The model under review builds one solid part; all positions refer to its coordinate system, in mm. Face numbers are marked on the shaded views. A direction names the side the tool comes from. Coordinates: 2 decimals unless noted, no trailing zeros. Loops run counter-clockwise (first coordinate to the right, second up) from the corner with the lowest first, then second, coordinate; pieces in that order, holes last. Notation, with made-up numbers: (20, 14) - (38, 14) arc R19 cw to (38, 38) - close; hole circle Ø9 at (-10.5, 54.25). An arc over 180 degrees is marked (long way). One line per item, written item: value. Start each with the question number.
1. Mouldability with a two-part tool opening along X and no side actions: class the marked faces 1, 2 and 3 as +X half, -X half, draft (parallel to the pull), parting line (faces both ways), or undercut.
2. For the marked faces 4, 5 and 6, list the 3-axis set-ups (+Z, -Z, +X, -X, +Y, -Y) from which the entire face can be reached by the end or side of a thin tool; tool diameter is ignored.
3. To check wall thickness, follow line 1 (X direction, y = 2.3, z = 0); line 2 (X direction, y = 0.8, z = 0); line 3 (Y direction, x = -3.5, z = -4.5). State the ranges of each line that lie inside material, in increasing order.
4. Insertion check: P1, Ø3.5, axis at x = 0, z = 0, coming from the -Y side; P2, Ø0.7, axis at x = -0.5, y = 10, coming from the -Z side; P3, Ø2, axis at x = 3, y = 10.5, coming from the +Z side. Each pin has a flat end and moves straight along its axis. Give the tip position at first contact, or say it passes through.
5. We need section A-A, the plane x = 0. Give the boundary of the cut face in (y, z), then the cut area to 3 significant figures.
6. We need section D-D, the plane z = 10.25. Give the boundary of the cut face in (x, y), then the cut area to 3 significant figures.
7. We need section B-B, the plane y = 5.75. Give the boundary of the cut face in (x, z).
8. We need section C-C, the plane z = -2.5. Give the boundary of the cut face in (x, y), then the cut area to 3 significant figures.
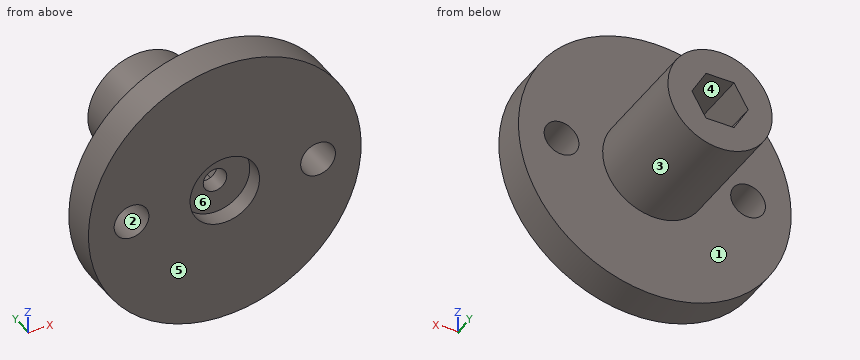
from build123d import *

# Parameters (mm, degrees)
SKETCH1_R           = 11.7729
SKETCH1_R_2         = 1.016
BOSS_EXTRUDE1_DEPTH = 3
SKETCH2_R           = 1.5
CUT_EXTRUDE1_DEPTH  = 17.917516036
SKETCH4_R           = 3
CUT_EXTRUDE3_DEPTH  = 1.5
SKETCH6_R           = 4.5
BOSS_EXTRUDE4_DEPTH = 10
CUT_EXTRUDE4_DEPTH  = 20.421697887


with BuildPart() as part:
    # Sketch1 → Boss-Extrude1 (new body)
    with BuildSketch(Plane(origin=(0, 0, 0), x_dir=(1, 0, 0), z_dir=(0, 1, 0))):
        with Locations(Location((0, 0, 0), (0, 0, 270))):
            Circle(SKETCH1_R)
        with Locations(Location((0, 0, 0), (0, 0, 270))):
            Circle(SKETCH1_R_2, mode=Mode.SUBTRACT)
    extrude(amount=BOSS_EXTRUDE1_DEPTH)

    # Sketch2 → Cut-Extrude1 (cut, through all)
    with BuildSketch(Plane(origin=(0, 3, 0), x_dir=(1, 0, 0), z_dir=(0, 1, 0))):
        with Locations(Location((8.0518, 0, 0), (0, 0, 270))):
            Circle(SKETCH2_R)
        with Locations(Location((-8.0518, 0, 0), (0, 0, 270))):
            Circle(SKETCH2_R)
    extrude(amount=-CUT_EXTRUDE1_DEPTH, mode=Mode.SUBTRACT)

    # Sketch4 → Cut-Extrude3 (cut)
    with BuildSketch(Plane.XZ):
        with Locations(Location((0, 0, 0), (0, 0, 270))):
            Circle(SKETCH4_R)
    extrude(amount=-CUT_EXTRUDE3_DEPTH, mode=Mode.SUBTRACT)

    # Sketch6 → Boss-Extrude4 (add)
    with BuildSketch(Plane(origin=(0, 3, 0), x_dir=(1, 0, 0), z_dir=(0, 1, 0))):
        with Locations(Location((0, 0, 0), (0, 0, 270))):
            Circle(SKETCH6_R)
    extrude(amount=BOSS_EXTRUDE4_DEPTH)

    # Sketch7 → Cut-Extrude4 (cut, through all)
    with BuildSketch(Plane.XZ.offset(-3)):
        Polygon((2.424871131, 0), (1.212435565, 2.1), (-1.212435565, 2.1), (-2.424871131, 0), (-1.212435565, -2.1), (1.212435565, -2.1), align=None)
    extrude(amount=-CUT_EXTRUDE4_DEPTH, mode=Mode.SUBTRACT)


solid = part.part
Findings below:
1. face 1: draft
1. face 2: undercut
1. face 3: parting line
2. face 4: +Y
2. face 5: +Z, -Z, +X, -X, -Y
2. face 6: -Y
3. line 1: -11.77 to -9.55, -6.55 to -1.02, 1.02 to 6.55, 9.55 to 11.77
3. line 2: -11.77 to -9.55, -6.55 to -3, 3 to 6.55, 9.55 to 11.77
3. line 3: 0 to 3
4. P1: y = 1.5
4. P2: z = -4.5
4. P3: z = 4.03
5. outline: (0, -11.77) - (3, -11.77) - (3, -4.5) - (13, -4.5) - (13, -2.1) - (3, -2.1) - (3, -1.02) - (1.5, -1.02) - (1.5, -3) - (0, -3) - close; (0, 3) - (1.5, 3) - (1.5, 1.02) - (3, 1.02) - (3, 2.1) - (13, 2.1) - (13, 4.5) - (3, 4.5) - (3, 11.77) - (0, 11.77) - close
5. area: 107 mm2
6. outline: (-5.79, 0) - (5.79, 0) - (5.79, 3) - (-5.79, 3) - close
6. area: 34.7 mm2
7. outline: circle Ø9 at (0, 0); hole (-2.42, 0) - (-1.21, -2.1) - (1.21, -2.1) - (2.42, 0) - (1.21, 2.1) - (-1.21, 2.1) - close
8. outline: (-11.5, 0) - (-1.66, 0) - (-1.66, 1.5) - (1.66, 1.5) - (1.66, 0) - (11.5, 0) - (11.5, 3) - (3.74, 3) - (3.74, 13) - (-3.74, 13) - (-3.74, 3) - (-11.5, 3) - close
8. area: 139 mm2
